from build123d import *

# Parameters (mm, degrees)
F0_W     = 75
F0_H     = 105
F1_DEPTH = 29
F2_W     = 7
F2_H     = 13
F3_DEPTH = 3
F6_DEPTH = 25
F7_R     = 5


with BuildPart() as f1:
    # F0 (on Front) → F1 (new body, symmetric)
    with BuildSketch(Plane.XZ):
        Rectangle(F0_W, F0_H)
        with BuildLine():
            Line((20.5, -7), (20.5, -18))
            Line((20.5, -18), (14.491377, -18))
            ThreePointArc((14.491377, -18), (0, -28), (-14.491377, -18))
            Line((-14.491377, -18), (-20.5, -18))
            Line((-20.5, -18), (-20.5, -7))
            Line((-20.5, -7), (-14.491377, -7))
            ThreePointArc((-14.491377, -7), (0, 3), (14.491377, -7))
            Line((14.491377, -7), (20.5, -7))
        make_face(mode=Mode.SUBTRACT)
    extrude(amount=F1_DEPTH, both=True)

    # F2 (on face) → F3 (join)
    with BuildSketch(Plane(origin=(0, 0, -52.5), x_dir=(1, 0, 0), z_dir=(0, 0, -1))):
        with Locations((-27.5, 35.5)):
            Rectangle(F2_W, F2_H)
        with Locations((27.5, -35.5)):
            Rectangle(F2_W, F2_H)
    extrude(amount=-F3_DEPTH)

    # F5 (on face) + F4 (on face) → F6 (cut)
    with BuildSketch(Plane.XY.offset(-49.5)):
        with BuildLine():
            Line((25.25, 42), (25.25, 36.5))
            ThreePointArc((25.25, 36.5), (27.5, 34.25), (29.75, 36.5))
            Line((29.75, 36.5), (29.75, 42))
            Line((29.75, 42), (25.25, 42))
        make_face()
    with BuildSketch(Plane.XY.offset(-49.5)):
        with BuildLine():
            Line((-25.25, -42), (-25.25, -36.5))
            ThreePointArc((-25.25, -36.5), (-27.5, -34.25), (-29.75, -36.5))
            Line((-29.75, -36.5), (-29.75, -42))
            Line((-29.75, -42), (-25.25, -42))
        make_face()
    extrude(amount=-F6_DEPTH, mode=Mode.SUBTRACT)

    # F7
    f7_edges = [f1.edges().sort_by_distance(p)[0] for p in [
        (-37.5, 0, -52.5),
        (37.5, 0, -52.5),
        (37.5, 0, 52.5),
        (-37.5, 0, 52.5),
    ]]
    fillet(f7_edges, radius=F7_R)


solid = f1.part
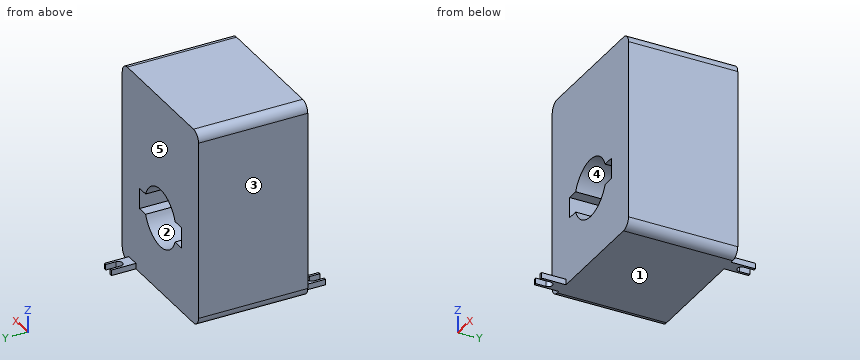
Input: part model. Units: mm. Frame: model coordinates. Face numbers are marked on the shaded views. A direction names the side the tool comes from. Coordinates: 2 decimals unless noted, no trailing zeros. Order: outer loops, then holes, each group sorted by start corner. A loop starts at its lowest first (then second) coordinate and runs counter-clockwise, first axis right, second up. Notation, with made-up numbers: M 62.5,85 L 101.5,85 A32 cw 101.5,115 Z; hole C -28,-12.75 d2. An arc over 180 degrees is marked long. Answer in a Markdown table with one row per item.
(1) Section query C-C, the plane y = -11. Output: boundary loops of the cut face in (x, z), plus the area to 3 significant figures.
Numbers:
| item | result |
|---|---|
| outline | M -37.5,-47.5 A5 ccw -32.5,-52.5 L 32.5,-52.5 A5 ccw 37.5,-47.5 L 37.5,47.5 A5 ccw 32.5,52.5 L -32.5,52.5 A5 ccw -37.5,47.5 Z; hole M -20.5,-18 L -14.49,-18 A15.5 ccw 14.49,-18 L 20.5,-18 L 20.5,-7 L 14.49,-7 A15.5 ccw -14.49,-7 L -20.5,-7 Z |
| area | 6,980 mm^2 |
(2) Contact query for flat-ended pins moving along their axis: pin 1 Ø1.5 at (x, z) = (-0.5, 37) entering from -Y; pin 2 Ø3.5 at (y, z) = (-36, -51) entering from -X; pin 3 Ø1.5 at (y, z) = (39, -51) entering from +X; pin 4 Ø8 at (y, z) = (31, -39.5) entering from -X. Output: stop coordinate, or through.
Numbers:
| item | result |
|---|---|
| pin 1 | stops at y = -29 |
| pin 2 | stops at x = -31 |
| pin 3 | stops at x = 31 |
| pin 4 | stops at x = -37.5 |
(3) Section query B-B, the plane x = 11. Output: boundary loops of the cut face in (y, z).
Numbers:
| item | result |
|---|---|
| outline | M -29,-52.5 L 29,-52.5 L 29,-23.42 L -29,-23.42 Z; M -29,-1.58 L 29,-1.58 L 29,52.5 L -29,52.5 Z |
(4) Access query for the marked faces 1 and 2. Directions: +Z, -Z, +X, -X, +Y, -Y. A direction counts if a zero-diameter tool reaches every point of the face in a straight line with its end or side. Return the directions, or none.
Numbers:
| item | result |
|---|---|
| face 1 | -Z, +X, -X, +Y, -Y |
| face 2 | +Y, -Y |
(5) Section query D-D, the plane x = -27.5. Output: boundary loops of the cut face in (y, z), plus the area to 3 significant figures.
Numbers:
| item | result |
|---|---|
| outline | M -34.25,-52.5 L 29,-52.5 L 29,52.5 L -29,52.5 L -29,-49.5 L -34.25,-49.5 Z |
| area | 6,110 mm^2 |
(6) Section query A-A, the plane z = -12. Output: boundary loops of the cut face in (x, y).
Numbers:
| item | result |
|---|---|
| outline | M -37.5,-29 L -20.5,-29 L -20.5,29 L -37.5,29 Z; M 20.5,-29 L 37.5,-29 L 37.5,29 L 20.5,29 Z |
(7) Material intervals for line 1 (Z direction, x = -17, y = 6); line 2 (Y direction, x = 20, z = -31.5); line 3 (X direction, y = 8, z = -13), sorted ascending. Write a range as [from, to].
Numbers:
| item | result |
|---|---|
| line 1 | z = [-52.5, -18], [-7, 52.5] |
| line 2 | y = [-29, 29] |
| line 3 | x = [-37.5, -20.5], [20.5, 37.5] |
(8) Draft query along X for the marked faces 3, 4 and 5. Return one class per face: pulls with the +X half, pulls with the -X half, needs draft (parallel to the pull), parting line crosses it, or undercut.
Numbers:
| item | result |
|---|---|
| face 3 | pulls with the -X half |
| face 4 | undercut |
| face 5 | needs draft |
